Autodesk Inventor part; units mm, degrees
ref_plane "YZ Plane" through (0, 0, 0) normal (1, 0, 0) x (0, 1, 0)
ref_plane "XZ Plane" through (0, 0, 0) normal (0, 1, 0) x (-1, 0, 0)
ref_plane "XY Plane" through (0, 0, 0) normal (0, 0, 1) x (1, 0, 0)
sketch "Sketch1" plane through (0, 0, 0) normal (0, 0, 1) x (1, 0, 0)
  line L0 (-12.552, 15.5925) -> (0.148, 15.5925)
  line L1 (0.148, 15.5925) -> (0.148, -9.8075)
  line L2 (0.148, -9.8075) -> (-12.552, -9.8075)
  line L3 (-12.552, -9.8075) -> (-12.552, 15.5925)
  point P0 (0, 0)
  dimension "d0" = 12.7
  dimension "d1" = 25.4
extrude "Extrusion1" add sketch "Sketch1" along normal blind 50.8
sketch "Sketch2" plane through (-12.552, 15.5925, 0) normal (0, 1, 0) x (1, 0, 0)
  line L0 (12.7, -50.8) -> (0, -50.8)
  line L1 (12.7, 0) -> (12.7, -50.8)
  point P0 (12.552, 0)
  point P1 (6.35, -38.1)
  point P2 (6.35, -12.7)
  dimension "d4" = 25.4
  dimension "d5" = 12.7
  dimension "d6" = 0
  dimension "d7" = 6.35
hole "Hole1" at (-6.202, 15.5925, 38.1) at (-6.202, 15.5925, 12.7) direction (0, -1, 0) diameter 3.175 end through all
sketch "Sketch3" plane through (0.148, -9.8075, 0) normal (1, 0, 0) x (0, 0, -1)
  line L0 (0, 0) -> (-50.8, 0)
  line L1 (0, 25.4) -> (-50.8, 25.4)
  line L2 (-50.8, 25.4) -> (0, 25.4)
  line L3 (0, 19.05) -> (-31.75, 0)
  line L4 (-31.75, 0) -> (-44.45, 0)
  line L5 (0, 0) -> (-50.8, 0)
  line L6 (-44.45, 0) -> (-50.8, 6.35)
  line L7 (-50.8, 0) -> (-44.3921, -0.0579)
  line L8 (-31.75, 0) -> (0, 0)
  line L9 (0, 19.05) -> (0, 0)
  line L10 (-50.8, 25.4) -> (-50.8, 0)
  line L11 (-50.8, 6.35) -> (-50.8, 0)
  point P0 (0, 9.8075)
  dimension "d18" = 12.7
  dimension "d19" = 19.05
  dimension "d20" = 6.35
extrude "Extrusion2" cut sketch "Sketch3" against normal blind 50.8
sketch "Sketch4" plane through (0, 0, 50.8) normal (0, 0, 1) x (1, 0, 0)
  line L0 (0.148, -9.8075) -> (-12.552, -9.8075)
  line L1 (-12.552, -9.8075) -> (-12.552, -3.4575)
  line L2 (0.148, -3.4575) -> (0.148, -9.8075)
  line L3 (-12.552, -3.4575) -> (0.148, -3.4575)
  line L4 (-12.552, -9.8075) -> (0.148, -9.8075)
  line L5 (-7.98, -9.8075) -> (-12.552, -9.8075)
  line L6 (-12.552, -9.8075) -> (-12.552, -3.4575)
  line L7 (-7.98, -9.8075) -> (-12.552, -3.4575)
  line L8 (0.148, -9.8075) -> (-4.805, -9.8075)
  line L9 (-4.805, -9.8075) -> (0.148, -3.4575)
  line L10 (0.148, -9.8075) -> (0.148, 9.2425)
  line L11 (0.148, -3.4575) -> (0.148, -9.8075)
  point P0 (0, 0)
  dimension "d23" = 3.175
  dimension "d24" = 4.572
  dimension "d25" = 4.953
extrude "Extrusion3" cut sketch "Sketch4" against normal blind 50.8 contours L0 L9 L2 | L0 L1 L7
properties part number "Slider"
For this review, take the finished solid that the model builds, in its own axes (mm). Coordinates: 2 decimals unless noted, no trailing zeros. Write each loop counter-clockwise with the first axis right and the second up, starting at its lowest first coordinate (ties: lowest second). Pieces come first, ordered by that corner, then holes. Notation, with made-up numbers: (32.5, 52.25) - (83.5, 52.25) arc R17 cw to (83.5, 82.25) - close; hole circle Ø1 at (77.5, 87). An arc over 180 degrees is marked (long way). Put each result on its own line as item: value.
1. Add section A-A, the plane x = -5.5. Give the boundary of the cut face in (y, z).
Values found:
outline: (-9.81, 31.75) - (0.77, 14.12) - (15.59, 14.12) - (15.59, 36.68) - (-9.81, 36.68) - close; (-9.81, 39.52) - (15.59, 39.52) - (15.59, 50.8) - (-3.46, 50.8) - (-9.81, 44.45) - close; (2.48, 11.28) - (9.24, 0) - (15.59, 0) - (15.59, 11.28) - close
2. For pin 1 (1 mm diameter, centred on x = -3, y = 5.5, fed in from -Z); pin 2 (6 mm diameter, centred on y = -4.5, z = 12.5, fed in from -X); pin 3 (2 mm diameter, centred on x = -10, y = -6, fed in from +Z); pin 4 (6 mm diameter, centred on x = -3.5, z = 11.5, fed in from -Y), all flat-tipped, find the tip position at first contact; note any pin that passes through.
Values found:
pin 1: z = 5.4
pin 2: through
pin 3: z = 49.26
pin 4: y = 0.54
3. Mouldability with a two-part tool opening along X and no side actions: class faces 1 (the flat face through (-1.81, -5.97, 36.19)), 2 (the cylindrical face through (-6.679, 8.027, 14.214)), 3 (the flat face through (-7.1, -9.808, 36.6)) as released by +X, released by -X, zero draft, split by the parting line, or undercut.
Values found:
face 1: released by +X
face 2: undercut
face 3: zero draft
4. Wall thickness on probe 1 along X at (y, z) = (9, 12.7); probe 2 along Z at (x, y) = (-5, 9.25); probe 3 along Z at (x, y) = (-7.5, -4.5): over which ranges is each line inside the solid? List them lowest first.
Values found:
probe 1: -12.55 to -7.79, -4.61 to 0.15
probe 2: 0 to 11.66, 13.74 to 37.06, 39.14 to 50.8
probe 3: 22.9 to 37.19, 39.01 to 49.76
5. Add section B-B, the plane z = 34. Give the boundary of the cut face in (x, y) (1 decimal), then the cut area to 3 significant figures.
Values found:
outline: (-12.6, -3.5) - (-8, -9.8) - (-4.8, -9.8) - (0.1, -3.5) - (0.1, 15.6) - (-12.6, 15.6) - close
area: 292 mm²
6. Add section C-C, the plane y = -5.5. Give the boundary of the cut face in (x, z) (1 decimal).
Values found:
outline: (-11.1, 24.6) - (-1.4, 24.6) - (-1.4, 48.8) - (-11.1, 48.8) - close; hole circle Ø3.2 at (-6.2, 38.1)
7. Add section D-D, the plane z = 12.7. Give the boundary of the cut face in (x, y).
Values found:
outline: (-12.55, 1.62) - (-7.79, 1.62) - (-7.79, 15.59) - (-12.55, 15.59) - close; (-4.61, 1.62) - (0.15, 1.62) - (0.15, 15.59) - (-4.61, 15.59) - close
